```python
from build123d import *

# Parameters (mm, degrees)
F0_W      = 44.703841
F0_H      = 67.055764
F1_DEPTH  = 25.4
F2_R      = 5.08
F3_R      = 4.871573
F4_DEPTH  = 58.928
F6_DEPTH  = 59.182
F7_R      = 3.027464
F8_DEPTH  = 69.85
F10_DEPTH = 63.246
F11_W     = 32.655392
F11_H     = 15.437096
F12_DEPTH = 55.372
F13_W     = 32.494774
F13_H     = 18.05481
F14_DEPTH = 12.192
F15_W     = 36.602098
F15_H     = 18.466117
F16_DEPTH = 9.398


with BuildPart() as f1:
    # F0 (on Front) → F1 (new body)
    with BuildSketch(Plane.XZ):
        with Locations((-7.164082, 23.068326)):
            Rectangle(F0_W, F0_H)
    extrude(amount=F1_DEPTH)

    # F2
    f2_edges = [f1.edges().sort_by_distance(p)[0] for p in [
        (-29.516002, -25.4, 23.068326),
        (15.187839, -25.4, 23.068326),
        (15.187839, 0, 23.068326),
        (-29.516002, 0, 23.068326),
    ]]
    fillet(f2_edges, radius=F2_R)

    # F3 (on Top) → F4 (join)
    with BuildSketch(Plane.XY):
        with Locations((-18.626601, -12.178931)):
            Circle(F3_R)
    extrude(amount=F4_DEPTH)

    # F5 (on Top) → F6 (join)
    with BuildSketch(Plane.XY):
        Polygon((-5.756941, -10.364093), (-5.343609, -16.772998), (0.413332, -19.619495), (5.756941, -16.057087), (5.343609, -9.648181), (-0.413332, -6.801685), align=None)
    extrude(amount=F6_DEPTH)

    # F7 (on Top) → F8 (cut)
    with BuildSketch(Plane.XY):
        with Locations((-18.405765, -11.726255)):
            Circle(F7_R)
    extrude(amount=F8_DEPTH, mode=Mode.SUBTRACT)

    # F9 (on Top) → F10 (cut)
    with BuildSketch(Plane.XY):
        Polygon((2.995406, -11.145309), (0, -9.415911), (-2.995406, -11.145309), (-2.995406, -14.604106), (0, -16.333505), (2.995406, -14.604106), align=None)
    extrude(amount=F10_DEPTH, mode=Mode.SUBTRACT)

    # F11 (on Top) → F12 (join)
    with BuildSketch(Plane.XY):
        with Locations((-6.234212, -13.507458)):
            Rectangle(F11_W, F11_H)
    extrude(amount=F12_DEPTH)

    # F13 (on Top) → F14 (cut)
    with BuildSketch(Plane.XY):
        with Locations((-6.848318, -12.28925)):
            Rectangle(F13_W, F13_H)
    extrude(amount=-F14_DEPTH, mode=Mode.SUBTRACT)

    # F15 (on Top) → F16 (join)
    with BuildSketch(Plane.XY):
        with Locations((-6.621592, -12.536748)):
            Rectangle(F15_W, F15_H)
    extrude(amount=-F16_DEPTH)


solid = f1.part
```
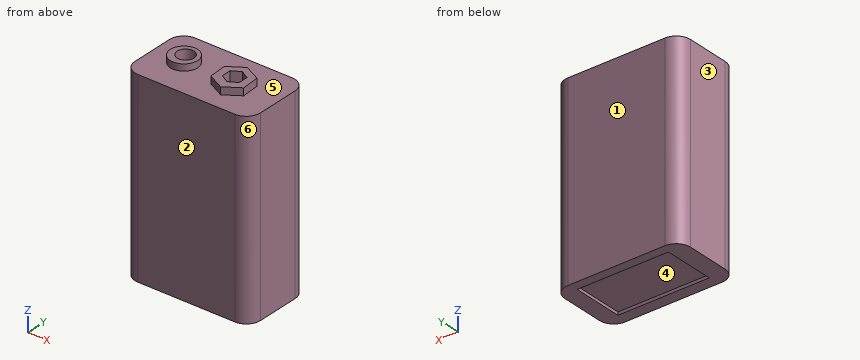
For this review, take the finished solid that the model builds, in its own axes (mm). Face numbers are marked on the shaded views. A direction names the side the tool comes from. Give positions to 0.01 mm unless a question says otherwise; leave off trailing zeros. Order: outer loops, then holes, each group sorted by start corner. A loop starts at its lowest first (then second) coordinate and runs counter-clockwise, first axis right, second up.
1) The part is to be moulded in two halves that separate along Y. For the marked faces 1, 2, 3 and 4, say which applies: released by +Y, released by -Y, zero draft, split by the parting line, or undercut.
2) Take a section at A-A (x = -8.5). Give the boundary of the cut face in (y, z), then the cut area to 3 significant figures.
3) Wall thickness on line 1 (Z direction, x = 13.5, y = -13); line 2 (Z direction, x = -13, y = -15); line 3 (X direction, y = -2, z = 43.5): over which ranges is each line inside the solid? List them lowest first.
4) Take a section at C-C (x = -4). Give the boundary of the cut face in (y, z), then the cut area to 3 significant figures.
5) Take a section at D-D (y = -1.25). Give the boundary of the cut face in (x, z), then the cut area to 3 significant figures.
6) Insertion check: pin 1 (1 mm diameter, centred on y = -12, z = 57.5, fed in from +X); pin 2 (3 mm diameter, centred on x = 0, y = -11.5, fed in from +Z); pin 3 (8 mm diameter, centred on x = -16.5, y = -11, fed in from +Z). Each pin has a flat end and moves straight along its axis. Give the tip position at first contact, or say it passes through.
7) For the marked faces 5 and 6, list the 3-axis set-ups (+Z, -Z, +X, -X, +Y, -Y) from which the entire face can be reached by the end or side of a thin tool; tool diameter is ignored.
8) Take a section at B-B (z = 28.5). Give the boundary of the cut face in (x, y), then the cut area to 3 significant figures.
Derived:
1. face 1: released by +Y
1. face 2: released by -Y
1. face 3: zero draft
1. face 4: undercut
2. outline: (-25.4, -10.46) - (-21.32, -10.46) - (-21.32, -9.4) - (-3.3, -9.4) - (-3.3, 0) - (-3.26, 0) - (-3.26, -10.46) - (0, -10.46) - (0, 56.6) - (-25.4, 56.6) - close
2. area: 1,680 mm2
3. line 1: z = -10.46 to 56.6
3. line 2: z = -9.4 to 56.6
3. line 3: x = -28.48 to 14.15
4. outline: (-25.4, -10.46) - (-21.32, -10.46) - (-21.32, -9.4) - (-3.3, -9.4) - (-3.3, 0) - (-3.26, 0) - (-3.26, -10.46) - (0, -10.46) - (0, 56.6) - (-9.19, 56.6) - (-9.19, 59.18) - (-17.44, 59.18) - (-17.44, 56.6) - (-25.4, 56.6) - close
4. area: 1,700 mm2
5. outline: (-27.77, -10.46) - (13.45, -10.46) - (13.45, 56.6) - (-27.77, 56.6) - close
5. area: 2,760 mm2
6. pin 1: stops at x = 5.53
6. pin 2: stops at z = 55.37
6. pin 3: stops at z = 58.93
7. face 5: +Z
7. face 6: +Z, -Z, +X, -Y
8. outline: (-29.52, -20.32) arc R5.08 ccw to (-24.44, -25.4) - (10.11, -25.4) arc R5.08 ccw to (15.19, -20.32) - (15.19, -5.08) arc R5.08 ccw to (10.11, 0) - (-24.44, 0) arc R5.08 ccw to (-29.52, -5.08) - close
8. area: 1,110 mm2
